from build123d import *

# Parameters (mm, degrees)
EXTRUDE_1_DEPTH     = 20
FILLET_1_R          = 9
SKETCH_2_R          = 2.55
CUT_EXTRUDE_1_DEPTH = 135.75780331
SKETCH_3_R          = 5
CUT_EXTRUDE_2_DEPTH = 6


with BuildPart() as part:
    # Эскиз1 → Бобышка-Вытянуть1 (new body)
    with BuildSketch(Plane(origin=(0, 0, 0), x_dir=(1, 0, 0), z_dir=(0, 1, 0))):
        with BuildLine():
            Line((-78.613569322, 20), (-53.613569322, 20))
            ThreePointArc((-53.613569322, 20), (-35.935899792, 12.67766953), (-28.613569322, -5))
            Line((-28.613569322, -5), (-28.613569322, -10))
            ThreePointArc((-28.613569322, -10), (-27.149103227, -13.535533906), (-23.613569322, -15))
            Line((-23.613569322, -15), (66.386430678, -15))
            ThreePointArc((66.386430678, -15), (69.921964584, -13.535533906), (71.386430678, -10))
            Line((71.386430678, -10), (71.386430678, -5))
            ThreePointArc((71.386430678, -5), (78.708761149, 12.67766953), (96.386430678, 20))
            Line((96.386430678, 20), (121.386430678, 20))
            Line((121.386430678, 20), (121.386430678, 15))
            ThreePointArc((121.386430678, 15), (116.993032396, 4.393398282), (106.386430678, 0))
            Line((106.386430678, 0), (98.386430678, 0))
            ThreePointArc((98.386430678, 0), (93.43668321, -2.050252532), (91.386430678, -7))
            Line((91.386430678, -7), (91.386430678, -15))
            ThreePointArc((91.386430678, -15), (85.528566302, -29.142135624), (71.386430678, -35))
            Line((71.386430678, -35), (-28.613569322, -35))
            ThreePointArc((-28.613569322, -35), (-42.755704945, -29.142135624), (-48.613569322, -15))
            Line((-48.613569322, -15), (-48.613569322, -7))
            ThreePointArc((-48.613569322, -7), (-50.663821853, -2.050252532), (-55.613569322, 0))
            Line((-55.613569322, 0), (-63.613569322, 0))
            ThreePointArc((-63.613569322, 0), (-74.220171039, 4.393398282), (-78.613569322, 15))
            Line((-78.613569322, 15), (-78.613569322, 20))
        make_face()
    extrude(amount=EXTRUDE_1_DEPTH)

    # Скругление1
    fillet_1_edges = [part.edges().sort_by_distance(p)[0] for p in [
        (-59.613569322, 20, 0),
        (-50.663821853, 20, 2.050252532),
        (-48.613569322, 20, 11),
        (-42.755704945, 20, 29.142135624),
        (21.386430678, 20, 35),
        (121.386430678, 0, -17.5),
        (116.993032396, 0, -4.393398282),
        (102.386430678, 0, 0),
        (93.43668321, 0, 2.050252532),
        (91.386430678, 0, 11),
        (85.528566302, 0, 29.142135624),
        (21.386430678, 0, 35),
        (85.528566302, 20, 29.142135624),
        (-42.755704945, 0, 29.142135624),
        (-48.613569322, 0, 11),
        (-50.663821853, 0, 2.050252532),
        (-59.613569322, 0, 0),
        (-74.220171039, 0, -4.393398282),
        (-78.613569322, 0, -17.5),
        (91.386430678, 20, 11),
        (93.43668321, 20, 2.050252532),
        (102.386430678, 20, 0),
        (116.993032396, 20, -4.393398282),
        (-78.613569322, 20, -17.5),
        (121.386430678, 20, -17.5),
        (-74.220171039, 20, -4.393398282),
    ]]
    fillet(fillet_1_edges, radius=FILLET_1_R)

    # Эскиз2 → Вырез-Вытянуть1 (cut, through all)
    with BuildSketch(Plane(origin=(0, 0, -20), x_dir=(-1, 0, 0), z_dir=(0, 0, -1))):
        with Locations((-111.386430678, 10)):
            Circle(SKETCH_2_R)
        with Locations((68.613569322, 10)):
            Circle(SKETCH_2_R)
    extrude(amount=-CUT_EXTRUDE_1_DEPTH, mode=Mode.SUBTRACT)

    # Эскиз3 → Вырез-Вытянуть2 (cut)
    with BuildSketch(Plane.XY):
        with Locations((-68.613569322, 10)):
            Circle(SKETCH_3_R)
        with Locations((111.386430678, 10)):
            Circle(SKETCH_3_R)
    extrude(amount=-CUT_EXTRUDE_2_DEPTH, mode=Mode.SUBTRACT)


solid = part.part
Build history of the part. All positions in model axes, mm. A direction names the side the tool comes from. Coordinates: 2 decimals unless noted, no trailing zeros. Order: outer loops, then holes, each group sorted by start corner. A loop starts at its lowest first (then second) coordinate and runs counter-clockwise, first axis right, second up. Notation, with made-up numbers: M 70.25,-12.5 L 82.25,-12.5 A32 ccw 82.25,26.5 Z; hole C 19,28.25 d7. An arc over 180 degrees is marked long. One line per question, with ' | ' between items. Start each with the question number.
Q1. Saw through at A-A (z = 12.5). List the corners of the cut face in (x, y).
Q2. Probe L1, parallel to X at y = 5, z = 10; L2, parallel to Y at x = 109, z = -5.5; L3, parallel to X at y = 16.5, z = 2. List the from-to ranges inside material, lowest first. Write a range as from..to.
Q3. Two-plate mould, pull along X, no slides. Class faces 6 (the face through (-77.24, 9.99, -8.73)), 7 (the face through (-28.614, 10, 7)), 8 (the face through (118.82, 2.706, -17.465)): +X half, -X half, draft (parallel to the pull), parting line (faces both ways), or undercut.
Q4. Flat gauge pins, fed straight in: pin 1 Ø4 at (y, z) = (11, 4.5) entering from +X; pin 2 Ø4 at (y, z) = (9.5, 6.5) entering from -X; pin 3 Ø1.6 at (y, z) = (10, 9) entering from -X; pin 4 Ø12 at (x, z) = (84.5, 11.5) entering from -Y. Where does each tip first touch, or does it go through?
Q5. 3-axis set-ups, long thin cutter, end or side, ignore diameter. For faces 1 (the face through (102.33, 17.294, -2.566)), 2 (the face through (88.82, 2.706, 11.056)), 3 (the face through (-27.188, 9.86, 13.496)), 4 (the face through (-59.67, 2.706, -2.566)), 5 (the face through (-59.67, 17.294, -2.566)): which of +Z, -Z, +X, -X, +Y, -Y reach the whole face in a straight line?
Q6. Saw through at B-B (x = 25.5). List the corners of the cut face in (y, z), then the cut area to 3 significant figures.
Check values:
1) outline: M -48.61,9 A9 ccw -39.61,0 L -27.94,0 L -27.94,20 L -39.61,20 A9 ccw -48.61,11 Z; M 70.72,0 L 82.39,0 A9 ccw 91.39,9 L 91.39,11 A9 ccw 82.39,20 L 70.72,20 Z
2) L1: x = -47.68..-28.61, 71.39..90.45 | L2: y = 0.87..5.61, 14.39..19.13 | L3: x = -48.28..-28.79, 71.57..91.05
3) face 6: -X half | face 7: undercut | face 8: +X half
4) pin 1: stops at x = 93.02 | pin 2: stops at x = -49.08 | pin 3: stops at x = -48.61 | pin 4: stops at y = 0
5) face 1: +Z, +X, +Y | face 2: +Z, +X, -Y | face 3: -Z, +Y, -Y | face 4: +Z, -X, -Y | face 5: +Z, -X, +Y
6) outline: M 0,15 L 20,15 L 20,26 A9 ccw 11,35 L 9,35 A9 ccw 0,26 Z | area: 365 mm2
